The listing builds one solid part. Answer for the finished solid, in the listing's coordinates (mm). A direction names the side the tool comes from. Give positions to 0.01 mm unless a question says otherwise; leave off trailing zeros. Order: outer loops, then holes, each group sorted by start corner. A loop starts at its lowest first (then second) coordinate and runs counter-clockwise, first axis right, second up. Notation, with made-up numbers: (82.25, 76) - (94.25, 76) arc R32 ccw to (94.25, 108) - close; hole circle Ø6 at (13, 23.5). An arc over 180 degrees is marked (long way). Answer in a Markdown table with one row per item. Add a question column.
```python
from build123d import *

# Parameters (mm, degrees)
PAD_DEPTH       = 15
SKETCH001_R     = 1.6
POCKET_DEPTH    = 8
SKETCH002_R     = 4
POCKET001_DEPTH = 3
FILLET_R        = 1
FILLET001_R     = 1
FILLET002_R     = 1
FILLET003_R     = 1
FILLET004_R     = 1
FILLET005_R     = 1
FILLET006_R     = 1
FILLET007_R     = 1
FILLET008_R     = 1
FILLET009_R     = 1
FILLET010_R     = 1
FILLET011_R     = 1
FILLET012_R     = 1
FILLET013_R     = 1
FILLET014_R     = 1
FILLET015_R     = 1


with BuildPart() as part:
    # Sketch → Pad (new body)
    with BuildSketch(Plane.XZ):
        Polygon((-30, 24.0033), (30, 24.0033), (30, 16.0033), (17, 16.0033), (17, -21.9967), (-30, -21.9967), (-30, -5.9967), (-26, -5.9967), (-26, -13.9967), (9, -13.9967), (9, 16.0033), (-30, 16.0033), align=None)
    extrude(amount=PAD_DEPTH)

    # Sketch001 → Pocket (cut)
    with BuildSketch(Plane(origin=(0, 0, 24.0033), x_dir=(-1, 0, 0), z_dir=(0, 0, 1))):
        with Locations((-24, 7.5)):
            Circle(SKETCH001_R)
        with Locations((24, 7.5)):
            Circle(SKETCH001_R)
    extrude(amount=-POCKET_DEPTH, mode=Mode.SUBTRACT)

    # Sketch002 → Pocket001 (cut)
    with BuildSketch(Plane(origin=(0, 0, 16.0033), x_dir=(1, 0, 0), z_dir=(0, 0, -1))):
        with Locations((24, 7.5)):
            Circle(SKETCH002_R)
        with Locations((-24, 7.5)):
            Circle(SKETCH002_R)
    extrude(amount=-POCKET001_DEPTH, mode=Mode.SUBTRACT)

    # Fillet
    fillet_edges = [part.edges().sort_by_distance(p)[0] for p in [
        (-8.5, -15, -13.9967),
    ]]
    fillet(fillet_edges, radius=FILLET_R)

    # Fillet001
    fillet001_edges = [part.edges().sort_by_distance(p)[0] for p in [
        (-26, -7.5, -5.9967),
    ]]
    fillet(fillet001_edges, radius=FILLET001_R)

    # Fillet002
    fillet002_edges = [part.edges().sort_by_distance(p)[0] for p in [
        (-30, -7.5, -5.9967),
    ]]
    fillet(fillet002_edges, radius=FILLET002_R)

    # Fillet003
    fillet003_edges = [part.edges().sort_by_distance(p)[0] for p in [
        (-30, -7.5, -21.9967),
    ]]
    fillet(fillet003_edges, radius=FILLET003_R)

    # Fillet004
    fillet004_edges = [part.edges().sort_by_distance(p)[0] for p in [
        (17, -7.5, -21.9967),
    ]]
    fillet(fillet004_edges, radius=FILLET004_R)

    # Fillet005
    fillet005_edges = [part.edges().sort_by_distance(p)[0] for p in [
        (-8.5, 0, -13.9967),
    ]]
    fillet(fillet005_edges, radius=FILLET005_R)

    # Fillet006
    fillet006_edges = [part.edges().sort_by_distance(p)[0] for p in [
        (17, -7.5, 16.0033),
    ]]
    fillet(fillet006_edges, radius=FILLET006_R)

    # Fillet007
    fillet007_edges = [part.edges().sort_by_distance(p)[0] for p in [
        (9, -7.5, 16.0033),
    ]]
    fillet(fillet007_edges, radius=FILLET007_R)

    # Fillet008
    fillet008_edges = [part.edges().sort_by_distance(p)[0] for p in [
        (-30, -7.5, 16.0033),
    ]]
    fillet(fillet008_edges, radius=FILLET008_R)

    # Fillet009
    fillet009_edges = [part.edges().sort_by_distance(p)[0] for p in [
        (30, -7.5, 16.0033),
    ]]
    fillet(fillet009_edges, radius=FILLET009_R)

    # Fillet010
    fillet010_edges = [part.edges().sort_by_distance(p)[0] for p in [
        (9, -15, 0.5033),
    ]]
    fillet(fillet010_edges, radius=FILLET010_R)

    # Fillet011
    fillet011_edges = [part.edges().sort_by_distance(p)[0] for p in [
        (9, 0, 0.5033),
    ]]
    fillet(fillet011_edges, radius=FILLET011_R)

    # Fillet012
    fillet012_edges = [part.edges().sort_by_distance(p)[0] for p in [
        (17, -15, -2.9967),
    ]]
    fillet(fillet012_edges, radius=FILLET012_R)

    # Fillet013
    fillet013_edges = [part.edges().sort_by_distance(p)[0] for p in [
        (17, 0, -2.9967),
    ]]
    fillet(fillet013_edges, radius=FILLET013_R)

    # Fillet014
    fillet014_edges = [part.edges().sort_by_distance(p)[0] for p in [
        (-28, -7.5, 19.0033),
    ]]
    fillet(fillet014_edges, radius=FILLET014_R)

    # Fillet015
    fillet015_edges = [part.edges().sort_by_distance(p)[0] for p in [
        (20, -7.5, 19.0033),
    ]]
    fillet(fillet015_edges, radius=FILLET015_R)


solid = part.part
```
(1) Each of these flat-tipped pins is pushed along its axis until it touches: P1, Ø6.5, axis at y = -6.5, z = -2.5, coming from the -X side; P2, Ø5.5, axis at y = -6, z = -9.5, coming from the +X side; P3, Ø8, axis at y = -1.5, z = -3, coming from the -X side; P4, Ø5.5, axis at x = 22, y = -7.5, coming from the -Z side. Where does it stop, or does it pass through?
(2) For faces 5 (the face through (-9, -7, -13.997)), 6 (the face through (-23.65, -5.94, 21.54)), 7 (the face through (20.8, -5.1, 17)), 8 (the face through (-10, -7, 16.003)), determine the directions among +Z, -Z, +X, -X, +Y, -Y from which every point of the face is accessible in a straight line to the end or side of a thin tool.
(3) Find section A-A, the plane x = -24. Write down the section's boundary in (y, z), plus the area to 3 significant figures.
(4) Find section C-C, the plane x = 24. Write down the section's boundary in (y, z).
(5) Find section D-D, the plane z = 7.5. Write down the section's boundary in (x, y).
(6) Straight lines are drawn through the part: line 1 (X direction, y = -7.5, z = 17.1); line 2 (X direction, y = -7.5, z = 20.8); line 3 (Y direction, x = 24, z = 17). For each, find the intervals that lie inside material, in ascending order.
(7) Find section B-B, the plane z = -9.5. Write down the section's boundary in (x, y), plus the area to 3 significant figures.
(8) The mould has two halves that part along X. Classify faces 1 (the face through (17, -7, -3)), 2 (the face through (25, -6, 19.003)), 3 (the face through (21.1, -4.5, 16.003)), 4 (the face through (-23, -6, 19.003)): +X half, -X half, draft (parallel to the pull), parting line (faces both ways), or undercut.
Answer key:
| question | item | result |
|---|---|---|
| 1 | P1 | x = 9 |
| 1 | P2 | x = 17 |
| 1 | P3 | x = -30 |
| 1 | P4 | z = 16 |
| 2 | face 5 | +Y, -Y |
| 2 | face 6 | +Z |
| 2 | face 7 | -Z |
| 2 | face 8 | -X, +Y, -Y |
| 3 | outline | (-15, -21) arc R1 ccw to (-14, -22) - (-1, -22) arc R1 ccw to (0, -21) - (0, -15) arc R1 ccw to (-1, -14) - (-14, -14) arc R1 ccw to (-15, -15) - close; (-15, 17) arc R1 ccw to (-14, 16) - (-11.5, 16) - (-11.5, 18) arc R1 cw to (-10.5, 19) - (-9.1, 19) - (-9.1, 24) - (-15, 24) - close; (-5.9, 19) - (-4.5, 19) arc R1 cw to (-3.5, 18) - (-3.5, 16) - (-1, 16) arc R1 ccw to (0, 17) - (0, 24) - (-5.9, 24) - close |
| 3 | area | 199 mm² |
| 4 | outline | (-15, 17) arc R1 ccw to (-14, 16) - (-11.5, 16) - (-11.5, 18) arc R1 cw to (-10.5, 19) - (-9.1, 19) - (-9.1, 24) - (-15, 24) - close; (-5.9, 19) - (-4.5, 19) arc R1 cw to (-3.5, 18) - (-3.5, 16) - (-1, 16) arc R1 ccw to (0, 17) - (0, 24) - (-5.9, 24) - close |
| 5 | outline | (9, -14) arc R1 ccw to (10, -15) - (16, -15) arc R1 ccw to (17, -14) - (17, -1) arc R1 ccw to (16, 0) - (10, 0) arc R1 ccw to (9, -1) - close |
| 6 | line 1 | -30 to -28, -20 to 20, 28 to 30 |
| 6 | line 2 | -30 to -25.6, -22.4 to 22.4, 25.6 to 30 |
| 6 | line 3 | -15 to -11.5, -3.5 to 0 |
| 7 | outline | (-30, -14) arc R1 ccw to (-29, -15) - (-27, -15) arc R1 ccw to (-26, -14) - (-26, -1) arc R1 ccw to (-27, 0) - (-29, 0) arc R1 ccw to (-30, -1) - close; (9, -14) arc R1 ccw to (10, -15) - (16, -15) arc R1 ccw to (17, -14) - (17, -1) arc R1 ccw to (16, 0) - (10, 0) arc R1 ccw to (9, -1) - close |
| 7 | area | 178 mm² |
| 8 | face 1 | +X half |
| 8 | face 2 | undercut |
| 8 | face 3 | draft |
| 8 | face 4 | undercut |
